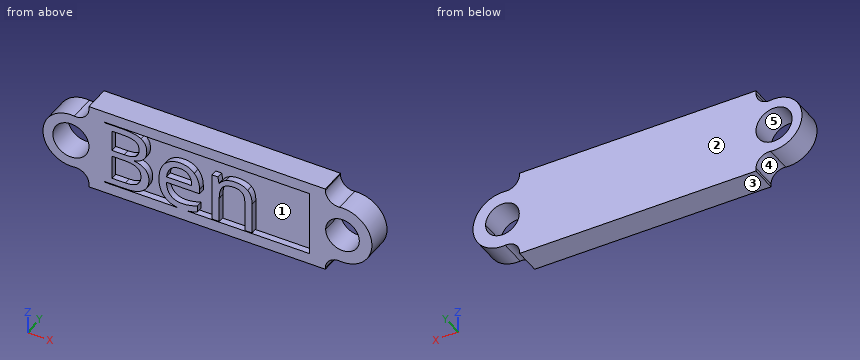
```python
from build123d import *

# Parameters (mm, degrees)
F0_R     = 17.5342485309
F0_W     = 208.0285698175
F0_H     = 60.8816854656
F1_DEPTH = 25.4
F2_W     = 199.1405338049
F2_H     = 63.4146874705
F3_DEPTH = 6.35
F6_DEPTH = 6.35


with BuildPart() as f1:
    # F0 (on Front) → F1 (new body)
    with BuildSketch(Plane.XZ):
        with BuildLine():
            Line((114.7961392999, 41.1091820392), (114.7961392999, 42.4124971032))
            Line((114.7961392999, 42.4124971032), (-114.7961392999, 42.4124971032))
            Line((-114.7961392999, 42.4124971032), (-114.7961392999, 39.5639197406))
            ThreePointArc((-114.7961392999, 39.5639197406), (-119.0780712792, 30.0546542169), (-129.0364748589, 26.9576765903))
            ThreePointArc((-129.0364748589, 26.9576765903), (-159.4885576846, 0), (-129.0364748589, -26.9576765903))
            ThreePointArc((-129.0364748589, -26.9576765903), (-119.0780712792, -30.0546542169), (-114.7961392999, -39.5639197406))
            Line((-114.7961392999, -39.5639197406), (-114.7961392999, -42.4124971032))
            Line((-114.7961392999, -42.4124971032), (114.7961392999, -42.4124971032))
            Line((114.7961392999, -42.4124971032), (114.7961392999, -41.1091820392))
            ThreePointArc((114.7961392999, -41.1091820392), (118.9582568629, -31.7073437353), (128.7165429996, -28.4679552471))
            ThreePointArc((128.7165429996, -28.4679552471), (160.0651957896, 0), (128.7165429996, 28.4679552471))
            ThreePointArc((128.7165429996, 28.4679552471), (118.9582568629, 31.7073437353), (114.7961392999, 41.1091820392))
        make_face()
        with Locations((-132.3303878307, 0)):
            Circle(F0_R, mode=Mode.SUBTRACT)
        Rectangle(F0_W, F0_H, mode=Mode.SUBTRACT)
        with BuildLine():
            ThreePointArc((115.1127634511, 0), (131.4648836851, 16.352120234), (147.8170039192, 0))
            ThreePointArc((147.8170039192, 0), (131.4648836851, -16.352120234), (115.1127634511, 0))
        make_face(mode=Mode.SUBTRACT)
        Rectangle(F0_W, F0_H)
    extrude(amount=F1_DEPTH)

    # F2 (on face) → F3 (cut)
    with BuildSketch(Plane.XZ.offset(25.4)):
        Rectangle(F2_W, F2_H)
    extrude(amount=-F3_DEPTH, mode=Mode.SUBTRACT)

    # F4 (on face) → F6 (join)
    with BuildSketch(Plane.XZ.offset(19.05)):
        with BuildLine():
            Line((36.5855240286, -0.8747291355), (36.5855240286, -31.0594588518))
            Line((36.5855240286, -31.0594588518), (43.6549620804, -31.0594588518))
            Line((43.6549620804, -31.0594588518), (43.6549620804, -0.6295463129))
            add(Edge.make_bspline(
                [(39.3983158546, 12.3855751871), (43.6549620804, 8.3196267123), (43.6549620804, -0.6295463129)],
                knots=[0, 0, 0, 1, 1, 1], degree=2))
            add(Edge.make_bspline(
                [(26.7101047848, 16.451523662), (35.1416696288, 16.451523662), (39.3983158546, 12.3855751871)],
                knots=[0, 0, 0, 1, 1, 1], degree=2))
            add(Edge.make_bspline(
                [(17.9856826804, 14.5513567868), (21.9017972081, 16.451523662), (26.7101047848, 16.451523662)],
                knots=[0, 0, 0, 1, 1, 1], degree=2))
            add(Edge.make_bspline(
                [(11.890165285, 9.2050091272), (14.0695681526, 12.6511899116), (17.9856826804, 14.5513567868)],
                knots=[0, 0, 0, 1, 1, 1], degree=2))
            Line((11.890165285, 9.2050091272), (11.549633587, 9.2050091272))
            Line((11.549633587, 9.2050091272), (10.4054470815, 15.5933837829))
            Line((10.4054470815, 15.5933837829), (4.6572720182, 15.5933837829))
            Line((4.6572720182, 15.5933837829), (4.6572720182, -31.0594588518))
            Line((4.6572720182, -31.0594588518), (11.72671007, -31.0594588518))
            Line((11.72671007, -31.0594588518), (11.72671007, -6.582040395))
            add(Edge.make_bspline(
                [(15.1320270506, 6.4875661767), (11.72671007, 2.5305878452), (11.72671007, -6.582040395)],
                knots=[0, 0, 0, 1, 1, 1], degree=2))
            add(Edge.make_bspline(
                [(25.8519649056, 10.4445445082), (18.5373440312, 10.4445445082), (15.1320270506, 6.4875661767)],
                knots=[0, 0, 0, 1, 1, 1], degree=2))
            add(Edge.make_bspline(
                [(33.9906724894, 7.6317526822), (31.3958209501, 10.4445445082), (25.8519649056, 10.4445445082)],
                knots=[0, 0, 0, 1, 1, 1], degree=2))
            add(Edge.make_bspline(
                [(36.5855240286, -0.8747291355), (36.5855240286, 4.8189608562), (33.9906724894, 7.6317526822)],
                knots=[0, 0, 0, 1, 1, 1], degree=2))
        make_face()
        with BuildLine():
            Line((-82.0965833805, 31.1761142863), (-99.5702669024, 31.1761142863))
            Line((-99.5702669024, 31.1761142863), (-99.5702669024, -31.0594588518))
            Line((-99.5702669024, -31.0594588518), (-77.9693392, -31.0594588518))
            add(Edge.make_bspline(
                [(-62.1959109457, -26.3737426865), (-67.8351158656, -31.0594588518), (-77.9693392, -31.0594588518)],
                knots=[0, 0, 0, 1, 1, 1], degree=2))
            add(Edge.make_bspline(
                [(-56.5567060258, -13.3518105525), (-56.5567060258, -21.6880265211), (-62.1959109457, -26.3737426865)],
                knots=[0, 0, 0, 1, 1, 1], degree=2))
            add(Edge.make_bspline(
                [(-70.7364459331, 1.5498565548), (-56.5567060258, -0.8747291355), (-56.5567060258, -13.3518105525)],
                knots=[0, 0, 0, 1, 1, 1], degree=2))
            Line((-70.7364459331, 1.5498565548), (-70.7364459331, 1.9721158604))
            add(Edge.make_bspline(
                [(-61.7259772024, 6.6305894899), (-64.8111943868, 3.0345747583), (-70.7364459331, 1.9721158604)],
                knots=[0, 0, 0, 1, 1, 1], degree=2))
            add(Edge.make_bspline(
                [(-58.6407600179, 15.7704602659), (-58.6407600179, 10.2266042214), (-61.7259772024, 6.6305894899)],
                knots=[0, 0, 0, 1, 1, 1], degree=2))
            add(Edge.make_bspline(
                [(-64.1778054284, 27.4711294114), (-58.6407600179, 23.7661445364), (-58.6407600179, 15.7704602659)],
                knots=[0, 0, 0, 1, 1, 1], degree=2))
            add(Edge.make_bspline(
                [(-82.0965833805, 31.1761142863), (-69.7148508389, 31.1761142863), (-64.1778054284, 27.4711294114)],
                knots=[0, 0, 0, 1, 1, 1], degree=2))
        make_face()
        with BuildLine():
            Line((-92.4487470017, -24.8890244829), (-92.4487470017, -1.5966563354))
            Line((-92.4487470017, -1.5966563354), (-80.0533931921, -1.5966563354))
            add(Edge.make_bspline(
                [(-68.2028900995, -4.3209099199), (-72.0985727254, -1.5966563354), (-80.0533931921, -1.5966563354)],
                knots=[0, 0, 0, 1, 1, 1], degree=2))
            add(Edge.make_bspline(
                [(-64.3072074737, -12.8342023714), (-64.3072074737, -7.0451635044), (-68.2028900995, -4.3209099199)],
                knots=[0, 0, 0, 1, 1, 1], degree=2))
            add(Edge.make_bspline(
                [(-68.114351858, -21.9740731475), (-64.3072074737, -19.0591218121), (-64.3072074737, -12.8342023714)],
                knots=[0, 0, 0, 1, 1, 1], degree=2))
            add(Edge.make_bspline(
                [(-79.4540574036, -24.8890244829), (-71.9214962424, -24.8890244829), (-68.114351858, -21.9740731475)],
                knots=[0, 0, 0, 1, 1, 1], degree=2))
            Line((-79.4540574036, -24.8890244829), (-92.4487470017, -24.8890244829))
        make_face(mode=Mode.SUBTRACT)
        with BuildLine():
            Line((-80.5301375694, 4.5329142298), (-92.4487470017, 4.5329142298))
            Line((-92.4487470017, 4.5329142298), (-92.4487470017, 24.9103310419))
            Line((-92.4487470017, 24.9103310419), (-81.7969154862, 24.9103310419))
            add(Edge.make_bspline(
                [(-69.878306054, 22.5947154951), (-73.6241547327, 24.9103310419), (-81.7969154862, 24.9103310419)],
                knots=[0, 0, 0, 1, 1, 1], degree=2))
            add(Edge.make_bspline(
                [(-66.1324573753, 15.0349117981), (-66.1324573753, 20.2790999483), (-69.878306054, 22.5947154951)],
                knots=[0, 0, 0, 1, 1, 1], degree=2))
            add(Edge.make_bspline(
                [(-69.4969105522, 6.9370680181), (-66.1324573753, 9.3412218065), (-66.1324573753, 15.0349117981)],
                knots=[0, 0, 0, 1, 1, 1], degree=2))
            add(Edge.make_bspline(
                [(-80.5301375694, 4.5329142298), (-72.861363729, 4.5329142298), (-69.4969105522, 6.9370680181)],
                knots=[0, 0, 0, 1, 1, 1], degree=2))
        make_face(mode=Mode.SUBTRACT)
        with BuildLine():
            add(Edge.make_bspline(
                [(-28.1770388712, -31.7073437353), (-35.9783446463, -30.7660762397), (-40.8718160129, -25.6109516828)],
                knots=[0.1825887008, 0.1825887008, 0.1825887008, 1, 1, 1], degree=2))
            Line((-28.1770388712, -31.7073437353), (-19.8087642709, -31.7073437353))
            add(Edge.make_bspline(
                [(-16.4829357976, -31.209292799), (-18.0019268098, -31.5316908913), (-19.8087642709, -31.7073437353)],
                knots=[0, 0, 0, 0.4551678559, 0.4551678559, 0.4551678559], degree=2))
            add(Edge.make_bspline(
                [(-9.3998764779, -28.8936772521), (-13.1457251566, -30.500986867), (-16.4829357976, -31.209292799)],
                knots=[0, 0, 0, 1, 1, 1], degree=2))
            Line((-9.3998764779, -28.8936772521), (-9.3998764779, -22.587030204))
            add(Edge.make_bspline(
                [(-24.2879223172, -25.7335430941), (-16.7553611561, -25.7335430941), (-9.3998764779, -22.587030204)],
                knots=[0, 0, 0, 1, 1, 1], degree=2))
            add(Edge.make_bspline(
                [(-35.3756344062, -21.4768968683), (-31.4390879766, -25.7335430941), (-24.2879223172, -25.7335430941)],
                knots=[0, 0, 0, 1, 1, 1], degree=2))
            add(Edge.make_bspline(
                [(-39.5301211226, -9.0066260852), (-39.3121808358, -17.2202506425), (-35.3756344062, -21.4768968683)],
                knots=[0, 0, 0, 1, 1, 1], degree=2))
            Line((-39.5301211226, -9.0066260852), (-7.3975500933, -9.0066260852))
            Line((-7.3975500933, -9.0066260852), (-7.3975500933, -4.5388502066))
            add(Edge.make_bspline(
                [(-12.5055255642, 10.6829166968), (-7.3975500933, 4.9143097316), (-7.3975500933, -4.5388502066)],
                knots=[0, 0, 0, 1, 1, 1], degree=2))
            add(Edge.make_bspline(
                [(-26.3719763094, 16.451523662), (-17.6135010352, 16.451523662), (-12.5055255642, 10.6829166968)],
                knots=[0, 0, 0, 1, 1, 1], degree=2))
            add(Edge.make_bspline(
                [(-41.3008859525, 9.8111555498), (-35.7434086401, 16.451523662), (-26.3719763094, 16.451523662)],
                knots=[0, 0, 0, 1, 1, 1], degree=2))
            add(Edge.make_bspline(
                [(-46.8583632649, -8.1212436702), (-46.8583632649, 3.1707874375), (-41.3008859525, 9.8111555498)],
                knots=[0, 0, 0, 1, 1, 1], degree=2))
            add(Edge.make_bspline(
                [(-40.8718160129, -25.6109516828), (-46.8583632649, -19.3043046347), (-46.8583632649, -8.1212436702)],
                knots=[0, 0, 0, 1, 1, 1], degree=2))
        make_face()
        with BuildLine():
            add(Edge.make_bspline(
                [(-26.4673251849, 10.5262721157), (-32.0792875689, 10.5262721157), (-35.4233088439, 6.8689616785)],
                knots=[0, 0, 0, 1, 1, 1], degree=2))
            add(Edge.make_bspline(
                [(-17.9472220993, 6.9711211879), (-20.9234691404, 10.5262721157), (-26.4673251849, 10.5262721157)],
                knots=[0, 0, 0, 1, 1, 1], degree=2))
            add(Edge.make_bspline(
                [(-14.9709750582, -3.2584510219), (-14.9709750582, 3.4159702601), (-17.9472220993, 6.9711211879)],
                knots=[0, 0, 0, 1, 1, 1], degree=2))
            Line((-14.9709750582, -3.2584510219), (-39.3666659075, -3.2584510219))
            add(Edge.make_bspline(
                [(-35.4233088439, 6.8689616785), (-38.7673301189, 3.2116512413), (-39.3666659075, -3.2584510219)],
                knots=[0, 0, 0, 1, 1, 1], degree=2))
        make_face(mode=Mode.SUBTRACT)
    extrude(amount=F6_DEPTH)


solid = f1.part
```
Verification items for the finished model (mm, model axes). Face numbers are marked on the shaded views. A direction names the side the tool comes from. Give positions to 0.01 mm unless a question says otherwise; leave off trailing zeros. Loops run counter-clockwise (first coordinate to the right, second up) from the corner with the lowest first, then second, coordinate; pieces in that order, holes last. Notation, with made-up numbers: M 61.25,-28 L 74.25,-28 A29 ccw 74.25,5 Z; hole C 30.5,-21 d1. An arc over 180 degrees is marked long. Return JSON: item names as keys, results as strings.
1) Section check A-A, the plane y = -11.25. Enter the section's corners in (x, z).
Findings:
{"outline": "M -129.04,-26.96 A12.7 cw -114.8,-39.56 L -114.8,-42.41 L 114.8,-42.41 L 114.8,-41.11 A12.7 cw 128.72,-28.47 A28.6 ccw long 128.72,28.47 A12.7 cw 114.8,41.11 L 114.8,42.41 L -114.8,42.41 L -114.8,39.56 A12.7 cw -129.04,26.96 A27.16 ccw long Z; hole C -132.33,0 d35.07; hole C 131.46,0 d32.7"}
2) Material ranges on L1, parallel to Z at x = -48.5, y = -21; L2, parallel to Z at x = 25, y = -20.75; L3, parallel to X at y = -11.25, z = -1.5, recorded low to high. Write a range as [from, to].
Findings:
{"L1": "z = [-42.41, -31.71], [31.71, 42.41]", "L2": "z = [-42.41, -31.71], [10.43, 16.39], [31.71, 42.41]", "L3": "x = [-159.45, -149.8], [-114.86, 115.18], [147.75, 160.03]"}
3) Tool access check on the marked faces 1 and 2. Record the directions out of +Z, -Z, +X, -X, +Y, -Y that give a thin tool (end or side, any length) a straight path to the whole face; none if there is none.
Findings:
{"face 1": "-Y", "face 2": "+Z, -Z, +X, -X, +Y"}
4) Section check B-B, the plane x = -137. Enter the section's corners in (y, z), and give its area (3 significant figures).
Findings:
{"outline": "M -25.4,-26.75 L 0,-26.75 L 0,-16.9 L -25.4,-16.9 Z; M -25.4,16.9 L 0,16.9 L 0,26.75 L -25.4,26.75 Z", "area": "501 mm2"}
5) Mould release check, pull along X, two halves, no side actions. Record for the marked faces 3, 4 and 5: released by +X, released by -X, zero draft, split by the parting line, or undercut.
Findings:
{"face 3": "zero draft", "face 4": "undercut", "face 5": "undercut"}
6) Gauge pin test, flat ends, axial feed: P1, Ø1, axis at x = 125, y = -18, coming from the -Z side; P2, Ø2, axis at y = -14, z = 33, coming from the -X side; P3, Ø1.9, axis at y = -22, z = -12, coming from the -X side. Record the tip position at first contact, or that the pin passes through.
Findings:
{"P1": "stops at z = -28.77", "P2": "stops at x = -117.29", "P3": "stops at x = -157.14"}
